from build123d import *

# Parameters (mm, degrees)
BOSS_EXTRUDE1_DEPTH      = 9.525
BOSS_EXTRUDE1_DEPTH_BACK = 9.525
SKETCH3_R                = 6.35
SKETCH3_R_2              = 3.2004
CHAMFER1_SIZE            = 0.31496


with BuildPart() as part:
    # Sketch3 → Boss-Extrude1 (new, two sides: drawn at the far end of the back side and taken through both)
    with BuildSketch(Plane.XY.offset(-BOSS_EXTRUDE1_DEPTH_BACK)):
        Circle(SKETCH3_R)
        Circle(SKETCH3_R_2, mode=Mode.SUBTRACT)
    extrude(amount=BOSS_EXTRUDE1_DEPTH + BOSS_EXTRUDE1_DEPTH_BACK)

    # Chamfer1
    chamfer1_edges = [part.edges().sort_by_distance(p)[0] for p in [
        (-6.35, 0, -9.525),
        (-3.2004, 0, -9.525),
        (-6.35, 0, 9.525),
        (-3.2004, 0, 9.525),
    ]]
    chamfer(chamfer1_edges, length=CHAMFER1_SIZE)


solid = part.part
Part model, mm, in its own coordinate system. Round coordinates to 2 decimals unless told otherwise and drop trailing zeros. Write each loop counter-clockwise with the first axis right and the second up, starting at its lowest first coordinate (ties: lowest second). Pieces come first, ordered by that corner, then holes. Notation, with made-up numbers: (11, 38) - (32, 38) arc R28 ccw to (32, 63) - close; hole circle Ø1 at (-1.75, 19.25). An arc over 180 degrees is marked (long way). Use CSV: the item, a comma, the result in double quotes.
Item 1: Pull direction Y, two halves, no side cores. Call faces 1 (the cylindrical face through (-2.54, -1.95, -0.13)), 2 (the cylindrical face through (-1.38, -6.2, -0.13)), 3 (the flat face through (3, -3, -9.525)): pulls with the +Y half, pulls with the -Y half, needs draft (parallel to the pull), parting line crosses it, or undercut.
Results list:
face 1,"undercut"
face 2,"parting line crosses it"
face 3,"needs draft"
Item 2: Slice it at A-A, the plane y = 0. Write the cut outline in (x, z) (3 decimals).
Results list:
outline,"(-6.35, -9.21) - (-6.035, -9.525) - (-3.515, -9.525) - (-3.2, -9.21) - (-3.2, 9.21) - (-3.515, 9.525) - (-6.035, 9.525) - (-6.35, 9.21) - close; (3.2, -9.21) - (3.515, -9.525) - (6.035, -9.525) - (6.35, -9.21) - (6.35, 9.21) - (6.035, 9.525) - (3.515, 9.525) - (3.2, 9.21) - close"
Item 3: Flat gauge pins, fed straight in: P1, Ø1, axis at y = -1, z = 2.5, coming from the -X side; P2, Ø1, axis at y = -3, z = -6.5, coming from the -X side; P3, Ø2, axis at x = 4, z = 4.5, coming from the -Y side; P4, Ø5, axis at x = 2.5, y = 0.5, coming from the +Z side (3 decimals). Where does each tip first touch, or does it go through?
Results list:
P1,"stops at x = -6.33"
P2,"stops at x = -5.84"
P3,"stops at y = -5.6"
P4,"stops at z = 9.525"
Item 4: Wall check: L1, parallel to Y at x = 0, z = 4.5; L2, parallel to Y at x = 2, z = -7.25; L3, parallel to X at y = -1.75, z = 7.5. Give the ranges that are in metal, low to high.
Results list:
L1,"y = -6.35 to -3.2, 3.2 to 6.35"
L2,"y = -6.03 to -2.5, 2.5 to 6.03"
L3,"x = -6.1 to -2.68, 2.68 to 6.1"
Item 5: Slice it at C-C, the plane z = 0. Write the cut outline in (x, y).
Results list:
outline,"circle Ø12.7 at (0, 0); hole circle Ø6.4 at (0, 0)"
